Autodesk Inventor part; units mm, degrees
ref_plane "YZ Plane" through (0, 0, 0) normal (1, 0, 0) x (0, 1, 0)
ref_plane "XZ Plane" through (0, 0, 0) normal (0, 1, 0) x (-1, 0, 0)
ref_plane "XY Plane" through (0, 0, 0) normal (0, 0, 1) x (1, 0, 0)
sketch "Эскиз1" plane through (0, 0, 0) normal (0, 1, 0) x (-1, 0, 0)
  arc A0 (11.1553, 1) -> (11.1553, -1) centre (0, 0) ccw
  line L0 (-15, 15) -> (-15, -15)
  line L1 (-15, 15) -> (0, 15)
  line L2 (-15, -15) -> (0, -15)
  line L3 (11.1553, 1) -> (14.9666, 1)
  line L4 (14.9666, -1) -> (11.1553, -1)
  arc A1 (0, -15) -> (14.5107, -3.8) centre (0, 0) ccw
  arc A2 (14.5107, 3.8) -> (0, 15) centre (0, 0) ccw
  line L5 (11.1553, -1) -> (21.1553, -1)
  line L6 (21.1553, -1) -> (21.1553, -3.8)
  line L7 (21.1553, -3.8) -> (14.5107, -3.8)
  line L8 (11.1553, 1) -> (21.1553, 1)
  line L9 (21.1553, 1) -> (21.1553, 3.8)
  line L10 (21.1553, 3.8) -> (14.5107, 3.8)
  point P0 (15, 0)
  dimension "d0" = 22.4
  dimension "d2" = 30
  dimension "d5" = 2.8
  dimension "d6" = 2.8
extrude "Выдавливание1" add sketch "Эскиз1" along normal blind 10
fillet "Сопряжение1" radius 4 4 edges at (-21.1553, 10, 2.4) (-21.1553, 10, -2.4) (-21.1553, 0, 2.4) (-21.1553, 0, -2.4)
sketch "Эскиз3" plane through (-14.5107, 0, 3.8) normal (0, 0, 1) x (1, 0, 0)
  arc A0 (-6.6446, 4) -> (-2.6446, 0) centre (-2.6446, 4) ccw
  line L0 (-2.6446, 0) -> (0, 0)
  line L1 (0, 0) -> (0, 10)
  line L2 (-2.6446, 10) -> (0, 10)
  arc A1 (-2.6446, 10) -> (-6.6446, 6) centre (-2.6446, 6) ccw
  line L3 (-6.6446, 4) -> (-6.6446, 6)
  line L4 (-6.6446, 5) -> (-3.1446, 5) construction
  point P0 (14.5107, 0)
  dimension "d20" = 3.5
hole "Отверстие2" at (-17.6553, 5, 3.8) direction (0, 0, -1) diameter 3 depth 8 tip angle 118
fillet "Сопряжение2" radius 2 2 edges at (15, 5, 15) (15, 5, -15)
chamfer "Фаска1" distance 1 angle 45 16 edges at (11.2, 10, 0) (11.2, 0, 0) (6.5, 10, 15) (14.4142, 10, 14.4142) (15, 10, 0) (14.4142, 10, -14.4142) (6.5, 10, -15) (-9.1652, 10, -11.8743) (-9.1652, 10, 11.8743) (6.5, 0, 15) (14.4142, 0, 14.4142) (15, 0, 0) (14.4142, 0, -14.4142) (6.5, 0, -15) (-9.1652, 0, -11.8743) (-9.1652, 0, 11.8743)
properties part number "BasicMount 22mm"
The model under review builds one solid part; all positions refer to its coordinate system, in mm. A direction names the side the tool comes from. Give positions to 0.01 mm unless a question says otherwise; leave off trailing zeros. Write each loop counter-clockwise with the first axis right and the second up, starting at its lowest first coordinate (ties: lowest second). Pieces come first, ordered by that corner, then holes. Notation, with made-up numbers: M 19.25,-18.75 L 43.25,-18.75 A21 ccw 43.25,-7.75 Z; hole C 14,18 d6. An arc over 180 degrees is marked long. Write item = value, one per line. Start each with the question number.
Q1. We need section D-D (y = 7). State the section outline as (x, z) points.
Q2. For line 1 (Z direction, x = 0, y = 1); line 2 (X direction, y = 5, z = -1.75); line 3 (X direction, y = 5, z = 3), list the stretches that pass through material, from the lowest coordinate up.
Q3. We need section B-B (z = 0). State the section outline as (x, y) points, plus the area to 3 significant figures.
Q4. We need section C-C (y = 1.5). State the section outline as (x, z) points, plus the area to 3 significant figures.
Q5. Clearance check with flat-ended pins moving along their axes: pin 1 (4 mm diameter, centred on x = -18.5, y = 4.5, fed in from -Z); pin 2 (4 mm diameter, centred on x = -17.66, y = 5, fed in from +Z); pin 3 (4 mm diameter, centred on y = 1.5, z = 0, fed in from -X). State where each tip first meets the part, or that it passes through.
Q6. Machinability: for faces 4 (the face through (-16, 5, -1)), 5 (the face through (-20.01, 1.2, 2.42)), which of the approach directions +Z, -Z, +X, -X, +Y, -Y give a long, thin tool a straight path to every point of the face, cutting with its end or side? Answer none if there is none.
Q7. Mouldability with a two-part tool opening along Z and no side actions: class faces 1 (the face through (-9, 5, -12)), 2 (the face through (-21.155, 5, 2)), 3 (the face through (11.36, 9.17, 0.49)) as released by +Z, released by -Z, zero draft, split by the parting line, or undercut.
Q8. We need section A-A (y = 5). State the section outline as (x, z) points.
Result set:
q1.outline = M -21.03,-3.8 L -14.51,-3.8 A15 ccw 0,-15 L 13,-15 A2 ccw 15,-13 L 15,13 A2 ccw 13,15 L 0,15 A15 ccw -14.51,3.8 L -21.03,3.8 L -21.03,1 L -11.16,1 A11.2 cw long -11.16,-1 L -21.03,-1 Z
q2.line_1 = -15 to -11.2, 11.2 to 15
q2.line_2 = -21.16 to -19.16, -16.16 to -11.06, 11.06 to 15
q2.line_3 = -21.16 to -19.16, -16.16 to -10.79, 10.79 to 15
q3.outline = M 11.2,1 L 12.2,0 L 14,0 L 15,1 L 15,9 L 14,10 L 12.2,10 L 11.2,9 Z
q3.area = 36.0 mm2
q4.outline = M -20.28,-3.8 L -14.51,-3.8 A15 ccw 0,-15 L 13,-15 A2 ccw 15,-13 L 15,13 A2 ccw 13,15 L 0,15 A15 ccw -14.51,3.8 L -20.28,3.8 L -20.28,1 L -11.16,1 A11.2 cw long -11.16,-1 L -20.28,-1 Z
q4.area = 431 mm2
q5.pin_1 = -3.8
q5.pin_2 = 3.8
q5.pin_3 = -21.08
q6.face_4 = -X, +Y, -Y
q6.face_5 = +Z, -Z, -X, -Y
q7.face_1 = released by -Z
q7.face_2 = zero draft
q7.face_3 = undercut
q8.outline = M -21.16,-3.8 L -19.16,-3.8 L -19.16,-1 L -21.16,-1 Z; M -21.16,1 L -19.16,1 L -19.16,3.8 L -21.16,3.8 Z; M -16.16,-3.8 L -14.51,-3.8 A15 ccw 0,-15 L 13,-15 A2 ccw 15,-13 L 15,13 A2 ccw 13,15 L 0,15 A15 ccw -14.51,3.8 L -16.16,3.8 L -16.16,1 L -11.16,1 A11.2 cw long -11.16,-1 L -16.16,-1 Z
